Answer from the drawing. Dimensions are ordinates in mm from the lowest x, y and z of the part. Give positions to 0.01 mm unless a question says otherwise; leave off trailing zeros. Order: outer loops, then holes, each group sorted by start corner. A loop starts at its lowest first (then second) coordinate and runs counter-clockwise, first axis right, second up.
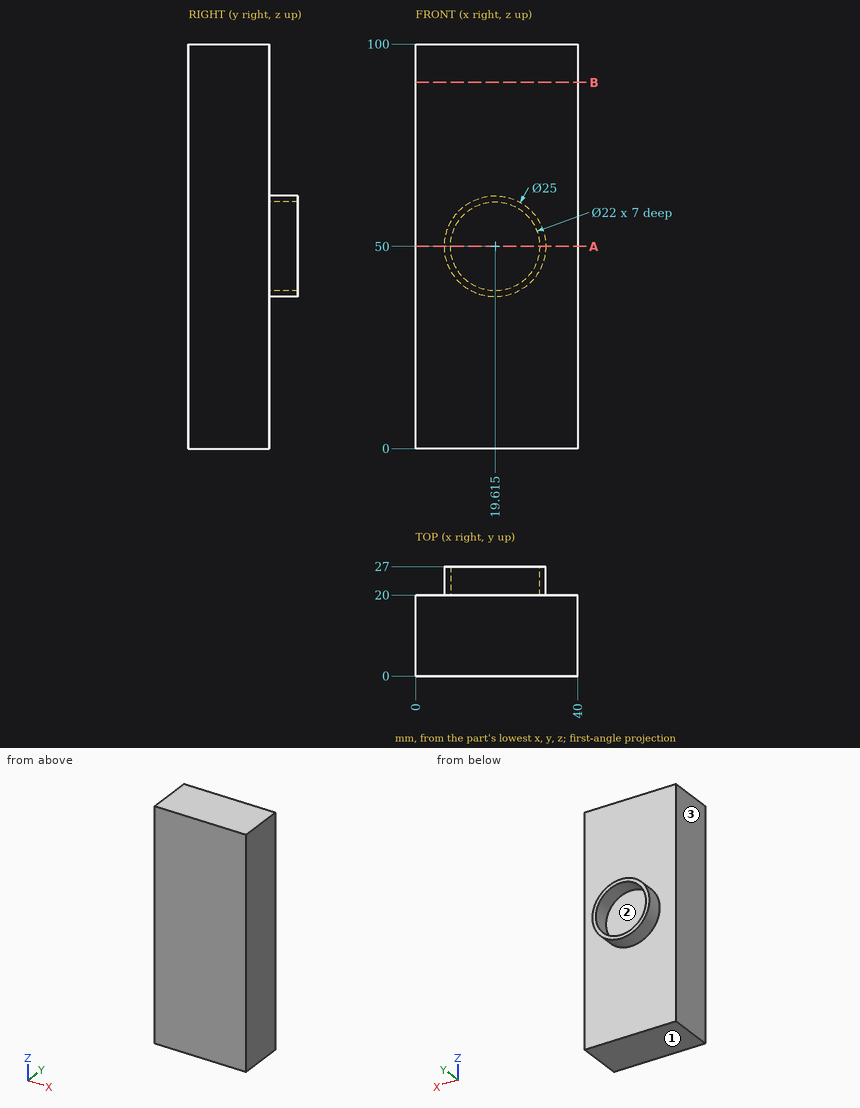
1. The mould has two halves that part along X. Classify the marked faces 1, 2 and 3: pulls with the +X half, pulls with the -X half, needs draft (parallel to the pull), parting line crosses it, or undercut.
Findings below:
face 1: needs draft
face 2: undercut
face 3: pulls with the -X half
2. The part is cut by section B-B (z = 90.5). Write down the section's boundary in (x, y).
Findings below:
outline: (0, 0) - (40, 0) - (40, 20) - (0, 20) - close
3. The part is cut by section A-A (z = 50). Write down the section's boundary in (x, y) (1 decimal).
Findings below:
outline: (0, 0) - (40, 0) - (40, 20) - (32.1, 20) - (32.1, 27) - (30.6, 27) - (30.6, 20) - (8.6, 20) - (8.6, 27) - (7.1, 27) - (7.1, 20) - (0, 20) - close
4. Given P1, Ø24, axis at x = 23, z = 47.5, coming from the +Y side; P2, Ø1.5, axis at x = 13.5, y = 21, coming from the +Z side; P3, Ø13, axis at x = 19.62, z = 50, coming from the +Y side, each flat-ended and moving along its own axis, determine where each tip first touches the part or whether it passes through.
Findings below:
P1: stops at y = 27
P2: stops at z = 61.29
P3: stops at y = 20
5. Straight lines are drawn through the part: probe 1 along X at (y, z) = (25, 50) (1 decimal); probe 2 along Y at (x, z) = (32, 75); probe 3 along Z at (x, y) = (14, 24.5). For each, find the intervals that lie inside material, in ascending order.
Findings below:
probe 1: x = 7.1 to 8.6, 30.6 to 32.1
probe 2: y = 0 to 20
probe 3: z = 38.83 to 40.54, 59.46 to 61.17
